from build123d import *

# Parameters (mm, degrees)
SKETCH1_W            = 77.75
SKETCH1_H            = 85
BOSS_EXTRUDE1_DEPTH  = 15.795
SKETCH2_W            = 82.2071
SKETCH2_H            = 98.425
BOSS_EXTRUDE2_DEPTH  = 5.588
M4_CLEARANCE_HOLE1_D = 4.5
CHAMFER1_SIZE        = 20
CHAMFER1_SIZE2       = 10
CHAMFER2_SIZE        = 10
CHAMFER2_SIZE2       = 20
CUT_EXTRUDE1_DEPTH   = 13.25
SKETCH7_W            = 4.4
SKETCH7_H            = 6.87
CUT_EXTRUDE2_DEPTH   = 68.5
SKETCH9_W            = 33.5
SKETCH9_H            = 11.5
CUT_EXTRUDE3_DEPTH   = 4.75
SKETCH10_W           = 9.4429
SKETCH10_H           = 6.99
CUT_EXTRUDE4_DEPTH   = 31.59
FILLET1_R            = 7.5
FILLET2_START        = -15.795
FILLET2_DEPTH        = 32.795
FILLET3_START        = -15.795
FILLET3_DEPTH        = 32.795
CHAMFER3_SIZE        = 5
CHAMFER3_SIZE2       = 20
SKETCH11_R           = 1.5
BOSS_EXTRUDE3_DEPTH  = 5


with BuildPart() as part:
    # Sketch1 → Boss-Extrude1 (new, symmetric)
    with BuildSketch(Plane(origin=(0, 0, 0), x_dir=(1, 0, 0), z_dir=(0, 1, 0))):
        Rectangle(SKETCH1_W, SKETCH1_H)
    extrude(amount=BOSS_EXTRUDE1_DEPTH, both=True)

    # Sketch2 → Boss-Extrude2 (add)
    with BuildSketch(Plane.XZ.offset(15.795)):
        with Locations((0, -4.8075)):
            Rectangle(SKETCH2_W, SKETCH2_H)
    extrude(amount=BOSS_EXTRUDE2_DEPTH)

    # M4 Clearance Hole1 (through all)
    with Locations(Plane(origin=(0, -21.383, 0), x_dir=(-1, 0, 0), z_dir=(0, -1, 0))):
        with Locations((-19.79355, 48.62), (19.79355, 48.62), (34.15355, -39.005), (-34.15355, -39.005)):
            Hole(M4_CLEARANCE_HOLE1_D / 2)

    # Chamfer1
    chamfer1_edges = [part.edges().sort_by_distance(p)[0] for p in [
        (41.10355, -18.589, -54.02),
    ]]
    chamfer1_side = [part.faces().sort_by_distance(p)[0] for p in [
        (0, -18.589, -54.02),
    ]]
    chamfer(chamfer1_edges, length=CHAMFER1_SIZE, length2=CHAMFER1_SIZE2, reference=chamfer1_side[0])

    # Chamfer2
    chamfer2_edges = [part.edges().sort_by_distance(p)[0] for p in [
        (-41.10355, -18.589, -54.02),
    ]]
    chamfer2_side = [part.faces().sort_by_distance(p)[0] for p in [
        (-41.10355, -18.589, -4.8075),
    ]]
    chamfer(chamfer2_edges, length=CHAMFER2_SIZE, length2=CHAMFER2_SIZE2, reference=chamfer2_side[0])

    # Sketch6 → Cut-Extrude1 (cut)
    with BuildSketch(Plane(origin=(0, 15.795, 0), x_dir=(1, 0, 0), z_dir=(0, 1, 0))):
        Polygon((-23.4, 42.5), (-23.4, 33.5), (-28.07, 33.5), (-28.07, 28.75), (-21.81, 16), (-19, 16), (-19, -26), (19, -26), (19, 16), (21.81, 16), (28.07, 28.75), (28.07, 33.5), (23.4, 33.5), (23.4, 42.5), align=None)
    extrude(amount=-CUT_EXTRUDE1_DEPTH, mode=Mode.SUBTRACT)

    # Sketch7 → Cut-Extrude2 (cut)
    with BuildSketch(Plane(origin=(0, 0, -42.5), x_dir=(-1, 0, 0), z_dir=(0, 0, -1))):
        with Locations((-21.2, 5.98)):
            Rectangle(SKETCH7_W, SKETCH7_H)
    cut_extrude2 = extrude(amount=-CUT_EXTRUDE2_DEPTH, mode=Mode.SUBTRACT)

    # Mirror7: Cut-Extrude2 across plane
    add(cut_extrude2.mirror(Plane(origin=(0, 0, 0), x_dir=(0, 0, 1), z_dir=(1, 0, 0))), mode=Mode.SUBTRACT)

    # Sketch9 → Cut-Extrude3 (cut)
    with BuildSketch(Plane(origin=(0, 15.795, 0), x_dir=(1, 0, 0), z_dir=(0, 1, 0))):
        with Locations((0, -31.75)):
            Rectangle(SKETCH9_W, SKETCH9_H)
    extrude(amount=-CUT_EXTRUDE3_DEPTH, mode=Mode.SUBTRACT)

    # Sketch10 → Cut-Extrude4 (cut)
    with BuildSketch(Plane(origin=(0, 15.795, 0), x_dir=(1, 0, 0), z_dir=(0, 1, 0))):
        with Locations((34.15355, -39.005)):
            Rectangle(SKETCH10_W, SKETCH10_H)
    cut_extrude4 = extrude(amount=-CUT_EXTRUDE4_DEPTH, mode=Mode.SUBTRACT)

    # Mirror8: Cut-Extrude4 across plane
    add(cut_extrude4.mirror(Plane(origin=(0, 0, 0), x_dir=(0, 0, 1), z_dir=(1, 0, 0))), mode=Mode.SUBTRACT)

    # Fillet1
    fillet1_edges = [part.edges().sort_by_distance(p)[0] for p in [
        (41.10355, -18.589, 44.405),
        (-41.10355, -18.589, 44.405),
        (38.875, 0, 35.51),
        (-38.875, 0, 35.51),
        (41.10355, -18.589, -44.02),
        (21.10355, -18.589, -54.02),
        (-21.10355, -18.589, -54.02),
        (-41.10355, -18.589, -44.02),
    ]]
    fillet(fillet1_edges, radius=FILLET1_R)

    # Fillet2: read off the stored shape, not the designer's step
    # Fillet2 outline → Fillet2 (cut)
    with BuildSketch(Plane(origin=(0, 0, 0), x_dir=(1, 0, 0), z_dir=(0, 1, 0)).offset(FILLET2_START)):
        with BuildLine():
            Line((-29.4321, -42.5), (-14.440772507, -42.5))
            add(Edge.make_bspline(
                [(-14.440772507, -42.5), (-29.194302513, -42.5), (-29.4321, -35.51)],
                knots=[0, 0, 0, 1, 1, 1], degree=2, weights=[1, 0.71902712, 1]))
            Line((-29.4321, -35.51), (-29.4321, -42.5))
        make_face()
    extrude(amount=FILLET2_DEPTH, mode=Mode.SUBTRACT)

    # Fillet3: read off the stored shape, not the designer's step
    # Fillet3 outline → Fillet3 (cut)
    with BuildSketch(Plane(origin=(0, 0, 0), x_dir=(1, 0, 0), z_dir=(0, 1, 0)).offset(FILLET3_START)):
        with BuildLine():
            add(Edge.make_bspline(
                [(14.440772507, -42.5), (29.194302513, -42.5), (29.4321, -35.51)],
                knots=[0, 0, 0, 1, 1, 1], degree=2, weights=[1, 0.71902712, 1]))
            Line((14.440772507, -42.5), (29.4321, -42.5))
            Line((29.4321, -42.5), (29.4321, -35.51))
        make_face()
    extrude(amount=FILLET3_DEPTH, mode=Mode.SUBTRACT)

    # Chamfer3
    chamfer3_edges = [part.edges().sort_by_distance(p)[0] for p in [
        (-31.1375, 15.795, -42.5),
    ]]
    chamfer3_side = [part.faces().sort_by_distance(p)[0] for p in [
        (30.40355, 15.795, 34.358042424),
    ]]
    chamfer(chamfer3_edges, length=CHAMFER3_SIZE, length2=CHAMFER3_SIZE2, reference=chamfer3_side[0])

    # Sketch11 → Boss-Extrude3 (add, symmetric)
    with BuildSketch(Plane.XY.offset(42.5)):
        with Locations(Location((-14.440772507, -11.383, 0), (0, 0, 270))):
            Circle(SKETCH11_R)
        with Locations(Location((14.440772507, -11.383, 0), (0, 0, 90))):
            Circle(SKETCH11_R)
    extrude(amount=BOSS_EXTRUDE3_DEPTH, both=True)


solid = part.part
Here's how the part is built. I have some questions about the finished solid (model axes, mm). A direction names the side the tool comes from. Give positions to 0.01 mm unless a question says otherwise; leave off trailing zeros. Loops run counter-clockwise (first coordinate to the right, second up) from the corner with the lowest first, then second, coordinate; pieces in that order, holes last. Notation, with made-up numbers: (84.25, -18.5) -> (92.25, -18.5) arc R22 cw to (92.25, -7.5) -> close; hole circle Ø2 at (6.25, 46.5). An arc over 180 degrees is marked (long way). Answer as a JSON object with one key per item and string values. Group by question number.
Item 1: I need wall thicknesses on L1, parallel to X at y = -17.6, z = -48.62; L2, parallel to X at y = 8, z = 0.5 (3 decimals); L3, parallel to X at y = -4.5, z = -20.5 (3 decimals). Which ranges of each line are inside material? Lowest first, please.
Item 2: Will these pins go through, and if not, where does the flat tip stop? pin 1 (7.5 mm diameter, centred on y = 4.5, z = 10.5, fed in from -X) (3 decimals); pin 2 (8 mm diameter, centred on x = -23, y = -8, fed in from -Z); pin 3 (1 mm diameter, centred on x = 4, y = 0.5, fed in from +Z); pin 4 (4 mm diameter, centred on x = 34.15, z = 39.01, fed in from +Y).
Item 3: On a 3-axis mill with a long thin cutter (end or side, diameter ignored), from which of +Z, -Z, +X, -X, +Y, -Y can I reach the whole of each face in a straight line? I mean faces 1 (the flat face through (23.4, 6, 3)), 2 (the flat face through (-25, 9.3, -22.5)), 3 (the cylindrical face through (-36.74, -0.22, 33.25)), 4 (the cylindrical face through (15.905, -11.708, 45.018)), 5 (the flat face through (-16.75, 13, 32)). Say none if no direction works.
Item 4: Thinking about a two-plate mould opening in X: for faces 6 (the flat face through (16.75, 13, 32)), 7 (the flat face through (29.92, -18.55, -49.61)), 8 (the cylindrical face through (-21.032, -18.628, -53.825)), which applies, pulls with the +X half, pulls with the -X half, needs draft (parallel to the pull), parting line crosses it, or undercut?
Item 5: Imagine slicing it at B-B on x = -9. Write out the boundary of the cut face in (y, z) (1 decimal).
Item 6: Imagine slicing it at A-A on z = -48.62. Write out the boundary of the cut face in (x, y) (3 decimals), then the cut area to 3 significant figures.
Answer list:
{
 "1": {"L1": "x = -31.9 to -22.04, -17.54 to 17.54, 22.04 to 31.9", "L2": "x = -38.875 to -23.4, 23.4 to 38.875", "L3": "x = -38.875 to 38.875"},
 "2": {"pin 1": "stops at x = -38.875", "pin 2": "stops at z = -42.5", "pin 3": "stops at z = 42.5", "pin 4": "passes through"},
 "3": {"face 1": "-Z", "face 2": "+Y", "face 3": "+Z, -X, +Y", "face 4": "+Z", "face 5": "-Z, +Y"},
 "4": {"face 6": "undercut", "face 7": "pulls with the +X half", "face 8": "pulls with the -X half"},
 "5": {"outline": "(-21.4, -54) -> (-15.8, -54) -> (-15.8, -42.5) -> (-4.2, -42.5) -> (2.5, -40.8) -> (2.5, 26) -> (11, 26) -> (11, 37.5) -> (15.8, 37.5) -> (15.8, 42.5) -> (-15.8, 42.5) -> (-15.8, 44.4) -> (-21.4, 44.4) -> close"},
 "6": {"outline": "(-31.904, -21.383) -> (-22.044, -21.383) -> (-22.044, -15.795) -> (-31.904, -15.795) -> close; (-17.544, -21.383) -> (17.544, -21.383) -> (17.544, -15.795) -> (-17.544, -15.795) -> close; (22.044, -21.383) -> (31.904, -21.383) -> (31.904, -15.795) -> (22.044, -15.795) -> close", "area": "306 mm2"}
}
